Here's how the part is built. I have some questions about the finished solid (model axes, mm). Face numbers are marked on the shaded views. A direction names the side the tool comes from. Round coordinates to 2 decimals unless told otherwise and drop trailing zeros. Loops run counter-clockwise (first coordinate to the right, second up) from the corner with the lowest first, then second, coordinate; pieces in that order, holes last. Notation, with made-up numbers: M 17.25,30 L 52.25,30 A23 ccw 52.25,50 Z; hole C 18.25,-30.75 d4. An arc over 180 degrees is marked long. Answer as a JSON object with one key per item and string values.
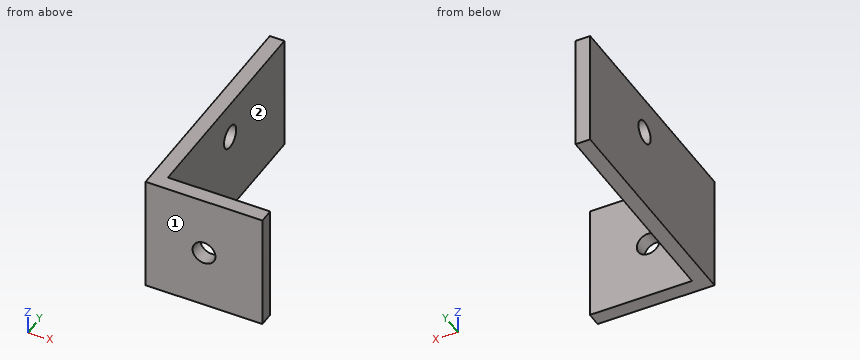
from build123d import *

# Parameters (mm, degrees)
BOSS_EXTRUDE1_DEPTH = 12.7
SKETCH2_R           = 2.4892
CUT_EXTRUDE1_DEPTH  = 56.448991199
SKETCH3_R           = 2.4892
CUT_EXTRUDE2_DEPTH  = 57.884801353


with BuildPart() as part:
    # Sketch1 → Boss-Extrude1 (new, symmetric)
    with BuildSketch(Plane.XY):
        Polygon((0, 0), (0, 50.8), (3.175, 50.8), (3.175, 3.175), (25.4, 3.175), (25.4, 0), align=None)
    extrude(amount=BOSS_EXTRUDE1_DEPTH, both=True)

    # Sketch2 → Cut-Extrude1 (cut, through all)
    with BuildSketch(Plane(origin=(0, 3.175, 0), x_dir=(1, 0, 0), z_dir=(0, 1, 0))):
        with Locations(Location((12.7, 0, 0), (0, 0, 180))):
            Circle(SKETCH2_R)
    extrude(amount=-CUT_EXTRUDE1_DEPTH, mode=Mode.SUBTRACT)

    # Sketch3 → Cut-Extrude2 (cut, through all)
    with BuildSketch(Plane(origin=(3.175, 0, 0), x_dir=(0, 0, -1), z_dir=(1, 0, 0))):
        with Locations(Location((-4.7625, 28.575, 0), (0, 0, 90))):
            Circle(SKETCH3_R)
    extrude(amount=-CUT_EXTRUDE2_DEPTH, mode=Mode.SUBTRACT)


solid = part.part
Item 1: I want a section at B-B on x = 12.7. List the corners of the cut face in (y, z) for me (3 decimals).
Solution:
{"outline": "M 0,-12.7 L 3.175,-12.7 L 3.175,-2.489 L 0,-2.489 Z; M 0,2.489 L 3.175,2.489 L 3.175,12.7 L 0,12.7 Z"}
Item 2: If I drill on L1, parallel to Z at x = 12.7, y = 1.95; L2, parallel to X at y = 25.5, z = -10.5 (3 decimals), over which ranges is the centre line in solid material (lowest first)? Write a range as from..to.
Solution:
{"L1": "z = -12.7..-2.49, 2.49..12.7", "L2": "x = 0..3.175"}
Item 3: For the marked faces 1 and 2, which set-ups out of +Z, -Z, +X, -X, +Y, -Y let a thin tool reach every point of the face, with its end or its side?
Solution:
{"face 1": "+Z, -Z, +X, -X, -Y", "face 2": "+Z, -Z, +X, +Y"}
Item 4: I want a section at C-C on y = 16. List the corners of the cut face in (x, z) for me (3 decimals).
Solution:
{"outline": "M 0,-12.7 L 3.175,-12.7 L 3.175,12.7 L 0,12.7 Z"}
Item 5: For P1, Ø8, axis at x = 15, z = -1, coming from the -Y side; P2, Ø1, axis at y = 35, z = -0.5, coming from the +X side (3 decimals); P3, Ø2, axis at x = 17, z = -1, coming from the +Y side (3 decimals), each with a flat end and sliding along its axis, tell me the tip position at first contact or that it passes through.
Solution:
{"P1": "stops at y = 0", "P2": "stops at x = 3.175", "P3": "stops at y = 3.175"}
Item 6: I want a section at A-A on z = 0. List the corners of the cut face in (x, y) for me (3 decimals).
Solution:
{"outline": "M 0,0 L 10.211,0 L 10.211,3.175 L 3.175,3.175 L 3.175,50.8 L 0,50.8 Z; M 15.189,0 L 25.4,0 L 25.4,3.175 L 15.189,3.175 Z"}
